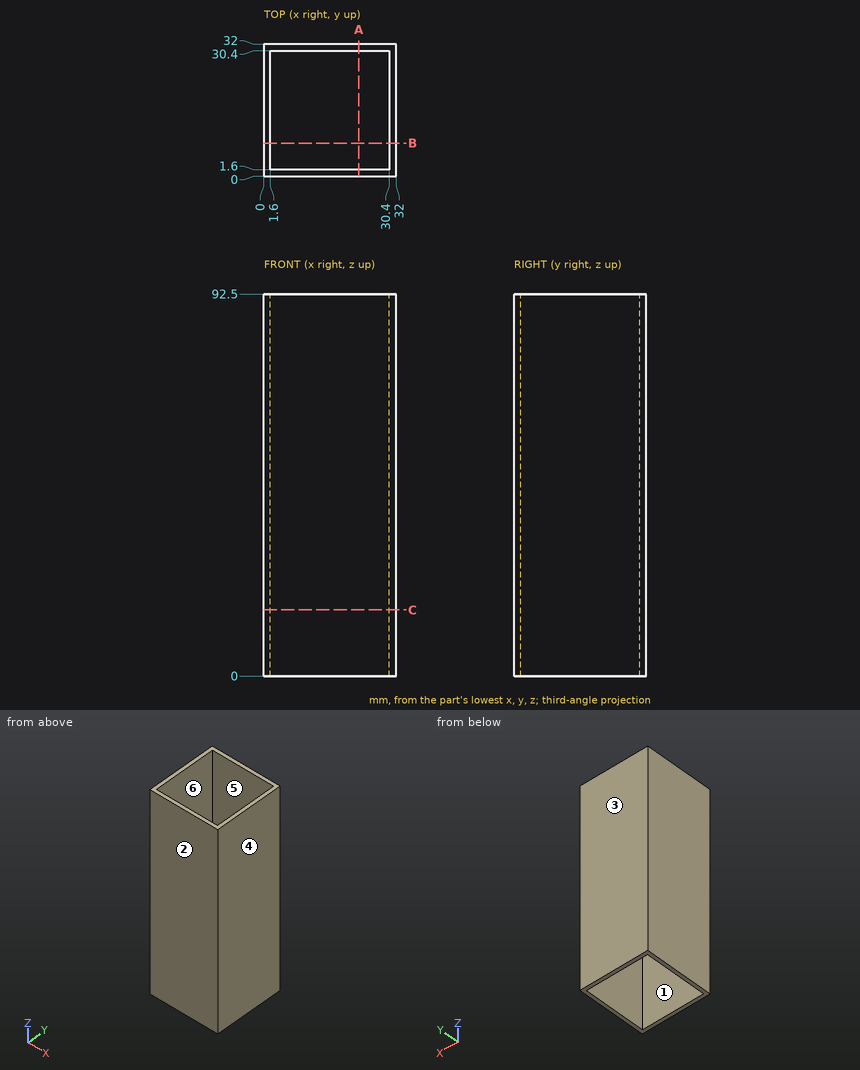
Geometry: see drawing. Coordinates: mm, zero at the bounding-box minimum. A direction names the side the tool comes from. Give positions to 0.01 mm unless a question says otherwise; leave off trailing zeros. Write each loop counter-clockwise with the first axis right and the second up, starting at its lowest first coordinate (ties: lowest second). Pieces come first, ordered by that corner, then holes. Notation, with made-up numbers: M 63,-31.5 L 75,-31.5 A3 ccw 75,-26.5 Z; hole C -30.5,-8 d11. An arc over 180 degrees is marked long. Return JSON: item names as keys, results as strings. Group by question number.
1) Draft query along X for the marked faces 3, 4, 5 and 6. Return one class per face: released by +X, released by -X, zero draft, split by the parting line, or undercut.
2) Cut plane A-A, the plane x = 23. Output: boundary loops of the cut face in (y, z).
3) Ray query, L1, parallel to X at y = 13, z = 32. Return the intervals inside material, ascending.
4) Cut plane C-C, the plane z = 16. Output: boundary loops of the cut face in (x, y).
5) First-contact query: pin 1 Ø8 at (y, z) = (10.5, 31.5) entering from -X. Flat tip, straight axial feed; report the tip coordinate or a pass-through.
6) Set-up query: the marked faces 1 and 2. Return all of +Z, -Z, +X, -X, +Y, -Y with unobstructed straight access to the full face (end or side cutting, diameter ignored); none if empty.
Data:
{
 "1": {"face 3": "zero draft", "face 4": "released by +X", "face 5": "undercut", "face 6": "undercut"},
 "2": {"outline": "M 0,0 L 1.6,0 L 1.6,92.5 L 0,92.5 Z; M 30.4,0 L 32,0 L 32,92.5 L 30.4,92.5 Z"},
 "3": {"L1": "x = 0 to 1.6, 30.4 to 32"},
 "4": {"outline": "M 0,0 L 32,0 L 32,32 L 0,32 Z; hole M 1.6,1.6 L 30.4,1.6 L 30.4,30.4 L 1.6,30.4 Z"},
 "5": {"pin 1": "stops at x = 0"},
 "6": {"face 1": "+Z, -Z", "face 2": "+Z, -Z, +X, -X, -Y"}
}
